Check sheet for the modelled part. Datum: model origin and axes. Units: mm. Round coordinates to 2 decimals unless told otherwise and drop trailing zeros. Loops run counter-clockwise (first coordinate to the right, second up) from the corner with the lowest first, then second, coordinate; pieces in that order, holes last. Notation, with made-up numbers: (86, 44) - (92, 44) arc R23 ccw to (92, 54) - close; hole circle Ø1 at (-36, 58). An arc over 180 degrees is marked (long way). Return JSON: item names as keys, results as strings.
from build123d import *

# Parameters (mm, degrees)
F0_R     = 2.38125
F1_DEPTH = 69.85
F2_R     = 3.175
F3_DEPTH = 0.79375
F4_R     = 0.396875


with BuildPart() as f1:
    # F0 (on Top) → F1 (new body)
    with BuildSketch(Plane.XY):
        Circle(F0_R)
    extrude(amount=F1_DEPTH)

    # F2 (on face) → F3 (join)
    with BuildSketch(Plane(origin=(0, 0, 0), x_dir=(1, 0, 0), z_dir=(0, 0, -1))):
        Circle(F2_R)
    extrude(amount=F3_DEPTH)

    # F4
    f4_edges = [f1.edges().sort_by_distance(p)[0] for p in [
        (-3.175, 0, -0.79375),
    ]]
    fillet(f4_edges, radius=F4_R)

    # F5: F1 across face


with BuildPart() as f1_1:
    add(f1.part)
    add(f1.part.mirror(Plane.XY.offset(69.85)))


solid = f1_1.part
Q1. Depth check by flat-ended pin: P1, Ø1.5, axis at y = -0.5, z = 107, coming from the +X side; P2, Ø3, axis at x = -1, z = 89, coming from the +Y side. Enter the tip coordinate at first touch or a pass-through.
Answer key:
{"P1": "stops at x = 2.38", "P2": "stops at y = 2.38"}
Q2. Scan lines: probe 1 along X at (y, z) = (-0.25, 23.5); probe 2 along Z at (x, y) = (2.5, -1). Record each from-to range of solid material in increasing order. Write a range as [from, to].
Answer key:
{"probe 1": "x = [-2.37, 2.37]", "probe 2": "z = [-0.79, 0], [139.7, 140.49]"}
Q3. Sectioned sample at C-C (z = 92). Enter the section's corners in (x, y), plus the area to 3 significant figures.
Answer key:
{"outline": "circle Ø4.76 at (0, 0)", "area": "17.8 mm²"}
Q4. Sectioned sample at A-A (x = 0). Enter the section's corners in (y, z) (3 decimals), plus the area to 3 significant figures.
Answer key:
{"outline": "(-3.175, -0.397) arc R0.397 ccw to (-2.778, -0.794) - (2.778, -0.794) arc R0.397 ccw to (3.175, -0.397) - (3.175, 0) - (2.381, 0) - (2.381, 139.7) - (3.175, 139.7) - (3.175, 140.097) arc R0.397 ccw to (2.778, 140.494) - (-2.778, 140.494) arc R0.397 ccw to (-3.175, 140.097) - (-3.175, 139.7) - (-2.381, 139.7) - (-2.381, 0) - (-3.175, 0) - close", "area": "675 mm²"}
